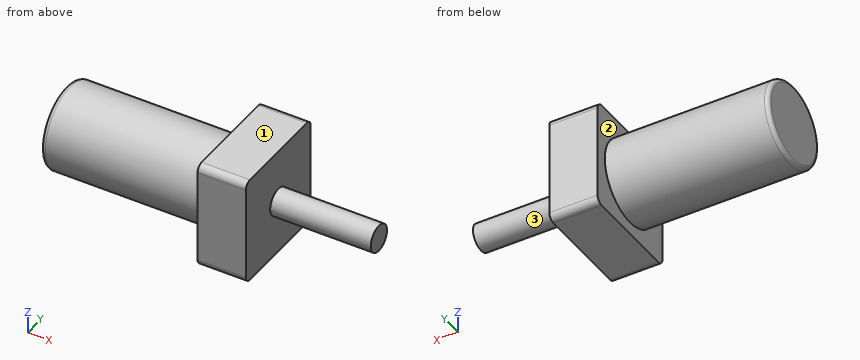
from build123d import *

# Parameters (mm, degrees)
SKETCH2_W           = 101.6
SKETCH2_H           = 101.6
BOSS_EXTRUDE1_DEPTH = 45.72
FILLET1_R           = 6.35
FILLET2_R           = 3.81


with BuildPart() as part:
    # Sketch1 → Revolve1 (revolve)
    with BuildSketch(Plane.XY):
        Polygon((154.94, 12.7), (295.91, 12.7), (295.91, 0), (0, 0), (0, 39.37), (154.94, 39.37), align=None)
    revolve(axis=Axis((-49.711428571, 0, 0), (1, 0, 0)))

    # Sketch2 → Boss-Extrude1 (add)
    with BuildSketch(Plane(origin=(154.94, 0, 0), x_dir=(0, 0, -1), z_dir=(1, 0, 0))):
        Rectangle(SKETCH2_W, SKETCH2_H)
    extrude(amount=BOSS_EXTRUDE1_DEPTH)

    # Fillet1
    fillet1_edges = [part.edges().sort_by_distance(p)[0] for p in [
        (177.8, 50.8, 50.8),
        (177.8, -50.8, 50.8),
        (177.8, -50.8, -50.8),
        (177.8, 50.8, -50.8),
    ]]
    fillet(fillet1_edges, radius=FILLET1_R)

    # Fillet2
    fillet2_edges = [part.edges().sort_by_distance(p)[0] for p in [
        (0, -39.37, 0),
    ]]
    fillet(fillet2_edges, radius=FILLET2_R)


solid = part.part
Read the model definition and answer for the solid it produces. Units are mm, in the model's axes. Face numbers are marked on the shaded views. A direction names the side the tool comes from. Coordinates: 2 decimals unless noted, no trailing zeros. Order: outer loops, then holes, each group sorted by start corner. A loop starts at its lowest first (then second) coordinate and runs counter-clockwise, first axis right, second up. Notation, with made-up numbers: M 16.5,32 L 44.5,32 A27 ccw 44.5,53 Z; hole C 82,79.5 d4. An arc over 180 degrees is marked long. Put each result on its own line as item: value. Start each with the question number.
Item 1: For the marked faces 1, 2 and 3, determine the directions among +Z, -Z, +X, -X, +Y, -Y from which every point of the face is accessible in a straight line to the end or side of a thin tool.
Item 2: Consider probe 1 along Z at (x, y) = (38.5, 0); probe 2 along X at (y, z) = (29, -45); probe 3 along X at (y, z) = (-21.5, -28). Determine where each line is inside the solid, lowest interval first. Write a range as [from, to].
Item 3: Section C-C, the plane x = 226.5 is taken. Determine the outline of the cut face in (y, z).
Item 4: Section D-D, the plane x = 83.5 is taken. Determine the outline of the cut face in (y, z).
Item 5: Given pin 1 Ø2 at (x, z) = (60.5, 24.5) entering from -Y; pin 2 Ø6 at (x, y) = (147, 35) entering from +Z; pin 3 Ø3 at (x, y) = (209.5, -9) entering from +Z, each flat-ended and moving along its own axis, determine where each tip first touches the part or whether it passes through.
Item 6: Section A-A, the plane y = 0 is taken. Determine the outline of the cut face in (x, z).
Computed:
1. face 1: +Z, +X, -X, +Y, -Y
1. face 2: -X
1. face 3: +X
2. probe 1: z = [-39.37, 39.37]
2. probe 2: x = [154.94, 200.66]
2. probe 3: x = [0, 200.66]
3. outline: C 0,0 d25.4
4. outline: C 0,0 d78.74
5. pin 1: stops at y = -31.59
5. pin 2: stops at z = 22.93
5. pin 3: stops at z = 10.25
6. outline: M 0,-35.56 A3.81 ccw 3.81,-39.37 L 154.94,-39.37 L 154.94,-50.8 L 200.66,-50.8 L 200.66,-12.7 L 295.91,-12.7 L 295.91,12.7 L 200.66,12.7 L 200.66,50.8 L 154.94,50.8 L 154.94,39.37 L 3.81,39.37 A3.81 ccw 0,35.56 Z
